```python
from build123d import *

# Parameters (mm, degrees)
SKETCH1_R      = 15
EXTRUDE1_DEPTH = 13
EXTRUDE2_START = -1.4
SKETCH2_R      = 15
SKETCH2_R_2    = 6
EXTRUDE2_DEPTH = 1.4
SKETCH3_R      = 1
EXTRUDE3_DEPTH = 4.4
SKETCH5_R      = 1
EXTRUDE5_DEPTH = 3
SKETCH6_R      = 2.5
EXTRUDE6_DEPTH = 25.879710609


with BuildPart() as part:
    # Sketch1 → Extrude1 (new body)
    with BuildSketch(Plane(origin=(0, 0, 0), x_dir=(1, 0, 0), z_dir=(0, 1, 0))):
        with Locations(Location((0, 0, 0), (0, 0, 90))):
            Circle(SKETCH1_R)
    extrude(amount=EXTRUDE1_DEPTH)

    # Sketch2 → Extrude2 (cut)
    with BuildSketch(Plane(origin=(0, 13, 0), x_dir=(1, 0, 0), z_dir=(0, 1, 0)).offset(EXTRUDE2_START)):
        with Locations(Location((0, 0, 0), (0, 0, 90))):
            Circle(SKETCH2_R)
        with Locations(Location((0, 0, 0), (0, 0, 270))):
            Circle(SKETCH2_R_2, mode=Mode.SUBTRACT)
    extrude(amount=EXTRUDE2_DEPTH, mode=Mode.SUBTRACT)

    # Sketch3 → Extrude3 (cut)
    with BuildSketch(Plane(origin=(0, 13, 0), x_dir=(1, 0, 0), z_dir=(0, 1, 0))):
        with Locations(Location((0, 12.7279, 0), (0, 0, 270))):
            Circle(SKETCH3_R)
        with Locations(Location((12.7279, 0, 0), (0, 0, 270))):
            Circle(SKETCH3_R)
        with Locations(Location((0, -12.7279, 0), (0, 0, 270))):
            Circle(SKETCH3_R)
        with Locations(Location((-12.7279, 0, 0), (0, 0, 270))):
            Circle(SKETCH3_R)
    extrude(amount=-EXTRUDE3_DEPTH, mode=Mode.SUBTRACT)

    # Sketch5 → Extrude5 (cut)
    with BuildSketch(Plane.XZ):
        with Locations(Location((-11, 5, 0), (0, 0, 270))):
            Circle(SKETCH5_R)
        with Locations(Location((11, 5, 0), (0, 0, 270))):
            Circle(SKETCH5_R)
        with Locations(Location((11, -5, 0), (0, 0, 270))):
            Circle(SKETCH5_R)
        with Locations(Location((-11, -5, 0), (0, 0, 270))):
            Circle(SKETCH5_R)
    extrude(amount=-EXTRUDE5_DEPTH, mode=Mode.SUBTRACT)

    # Sketch6 → Extrude6 (cut, through all)
    with BuildSketch(Plane.XZ):
        with Locations(Location((0, 0, 0), (0, 0, 270))):
            Circle(SKETCH6_R)
    extrude(amount=-EXTRUDE6_DEPTH, mode=Mode.SUBTRACT)


solid = part.part
```
The model under review builds one solid part; all positions refer to its coordinate system, in mm. A direction names the side the tool comes from. Round coordinates to 2 decimals unless told otherwise and drop trailing zeros. Order: outer loops, then holes, each group sorted by start corner. A loop starts at its lowest first (then second) coordinate and runs counter-clockwise, first axis right, second up.
Item 1: Add section D-D, the plane y = 12. State the section outline as (x, z) points.
Working result:
outline: circle Ø12 at (0, 0); hole circle Ø5 at (0, 0)
Item 2: For pin 1 (2 mm diameter, centred on x = -10.5, z = 5.5, fed in from -Y); pin 2 (2 mm diameter, centred on y = 9, z = 3, fed in from +X); pin 3 (4 mm diameter, centred on x = 7, z = -8, fed in from +Y); pin 4 (0.6 mm diameter, centred on x = -11, z = -5.5, fed in from -Y), all flat-tipped, find the tip position at first contact; note any pin that passes through.
Working result:
pin 1: stops at y = 0
pin 2: stops at x = 14.87
pin 3: stops at y = 11.6
pin 4: stops at y = 3
Item 3: Machinability: for faces 4 (the cylindrical face through (-13.704, 10.121, -0.217)), 5 (the flat face through (-11, 3, 5)), 6 (the cylindrical face through (-2.44, 6.41, 0.54)), which of the approach directions +Z, -Z, +X, -X, +Y, -Y give a long, thin tool a straight path to every point of the face, cutting with its end or side? Answer none if there is none.
Working result:
face 4: +Y
face 5: -Y
face 6: +Y, -Y
Item 4: Add section B-B, the plane x = 0. State the section outline as (y, z) points.
Working result:
outline: (0, -15) - (11.6, -15) - (11.6, -13.73) - (8.6, -13.73) - (8.6, -11.73) - (11.6, -11.73) - (11.6, -6) - (13, -6) - (13, -2.5) - (0, -2.5) - close; (0, 2.5) - (13, 2.5) - (13, 6) - (11.6, 6) - (11.6, 11.73) - (8.6, 11.73) - (8.6, 13.73) - (11.6, 13.73) - (11.6, 15) - (0, 15) - close
Item 5: Draft analysis for pull direction X (two halves, no side actions). For faces 1 (the cylindrical face through (10.4, 1.5, -4.2)), 2 (the flat face through (6.5, 11.6, 0.2)), 3 (the cylindrical face through (-0.66, 5.719, 14.985)), state which applies: released by +X, released by -X, zero draft, split by the parting line, or undercut.
Working result:
face 1: undercut
face 2: zero draft
face 3: split by the parting line
Item 6: To check wall thickness, follow probe 1 along X at (y, z) = (9.85, 0); probe 2 along X at (y, z) = (6.25, 0); probe 3 along Y at (x, z) = (6, -11.25). State the ranges of each line that lie inside material, in increasing order.
Working result:
probe 1: x = -15 to -13.73, -11.73 to -2.5, 2.5 to 11.73, 13.73 to 15
probe 2: x = -15 to -2.5, 2.5 to 15
probe 3: y = 0 to 11.6
Item 7: Add section C-C, the plane y = 2.25. State the section outline as (x, z) points, and give its area (3 significant figures).
Working result:
outline: circle Ø30 at (0, 0); hole circle Ø2 at (-11, -5); hole circle Ø2 at (-11, 5); hole circle Ø5 at (0, 0); hole circle Ø2 at (11, -5); hole circle Ø2 at (11, 5)
area: 675 mm2
Item 8: Add section A-A, the plane z = 0. State the section outline as (x, y) points.
Working result:
outline: (-15, 0) - (-2.5, 0) - (-2.5, 13) - (-6, 13) - (-6, 11.6) - (-11.73, 11.6) - (-11.73, 8.6) - (-13.73, 8.6) - (-13.73, 11.6) - (-15, 11.6) - close; (2.5, 0) - (15, 0) - (15, 11.6) - (13.73, 11.6) - (13.73, 8.6) - (11.73, 8.6) - (11.73, 11.6) - (6, 11.6) - (6, 13) - (2.5, 13) - close
